Can you work these out from the drawing? Everything is in mm from the part's minimum corner. Round coordinates to 2 decimals unless told otherwise and drop trailing zeros. Loops run counter-clockwise (first coordinate to the right, second up) from the corner with the lowest first, then second, coordinate; pieces in that order, holes last. Notation, with made-up numbers: (37.5, 79.5) -> (58.5, 79.5) arc R18 ccw to (58.5, 113.5) -> close; hole circle Ø1 at (58.5, -39). An arc over 180 degrees is marked (long way). Answer as a JSON object with one key per item and string values.
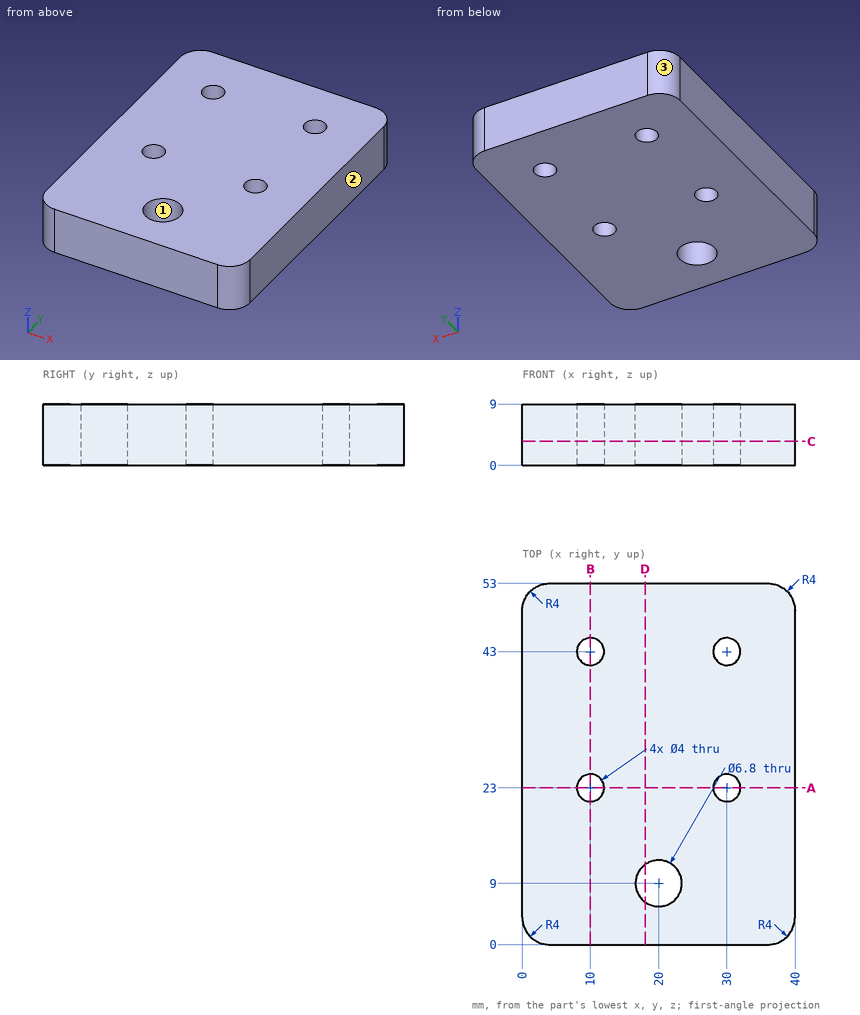
Q1. If I drill on L1, parallel to Y at x = 10, z = 3.5; L2, parallel to Y at x = 20, z = 2; L3, parallel to Y at x = 30.5, z = 2.75, over which ranges is the centre line in solid material (lowest first)? Write a range as [from, to].
Determined:
{"L1": "[0, 21], [25, 41], [45, 53]", "L2": "[0, 5.6], [12.4, 53]", "L3": "[0, 21.06], [24.94, 41.06], [44.94, 53]"}
Q2. I want a section at A-A, the plane y = 23. Write out the boundary of the cut face in (x, z).
Determined:
{"outline": "(0, 0) -> (8, 0) -> (8, 9) -> (0, 9) -> close; (12, 0) -> (28, 0) -> (28, 9) -> (12, 9) -> close; (32, 0) -> (40, 0) -> (40, 9) -> (32, 9) -> close"}
Q3. We'd pull the mould along X, two halves only. Please class the marked faces 1, 2 and 3: pulls with the +X half, pulls with the -X half, needs draft (parallel to the pull), parting line crosses it, or undercut.
Determined:
{"face 1": "undercut", "face 2": "pulls with the +X half", "face 3": "pulls with the -X half"}
Q4. I want a section at C-C, the plane z = 3.5. Write out the boundary of the cut face in (x, y), then the cut area to 3 significant figures.
Determined:
{"outline": "(0, 4) arc R4 ccw to (4, 0) -> (36, 0) arc R4 ccw to (40, 4) -> (40, 49) arc R4 ccw to (36, 53) -> (4, 53) arc R4 ccw to (0, 49) -> close; hole circle Ø4 at (10, 23); hole circle Ø4 at (10, 43); hole circle Ø6.8 at (20, 9); hole circle Ø4 at (30, 23); hole circle Ø4 at (30, 43)", "area": "2,020 mm²"}
Q5. I want a section at B-B, the plane x = 10. Write out the boundary of the cut face in (y, z), then the cut area to 3 significant figures.
Determined:
{"outline": "(0, 0) -> (21, 0) -> (21, 9) -> (0, 9) -> close; (25, 0) -> (41, 0) -> (41, 9) -> (25, 9) -> close; (45, 0) -> (53, 0) -> (53, 9) -> (45, 9) -> close", "area": "405 mm²"}
Q6. I'm going to push a flat-ended pin straight in: pin 1 (3 mm diameter, centred on x = 30, y = 43, fed in from -Z). Where does the tip first touch, or does it pass through?
Determined:
{"pin 1": "through"}
Q7. I want a section at D-D, the plane x = 18. Write out the boundary of the cut face in (y, z), then the cut area to 3 significant figures.
Determined:
{"outline": "(0, 0) -> (6.25, 0) -> (6.25, 9) -> (0, 9) -> close; (11.75, 0) -> (53, 0) -> (53, 9) -> (11.75, 9) -> close", "area": "428 mm²"}
